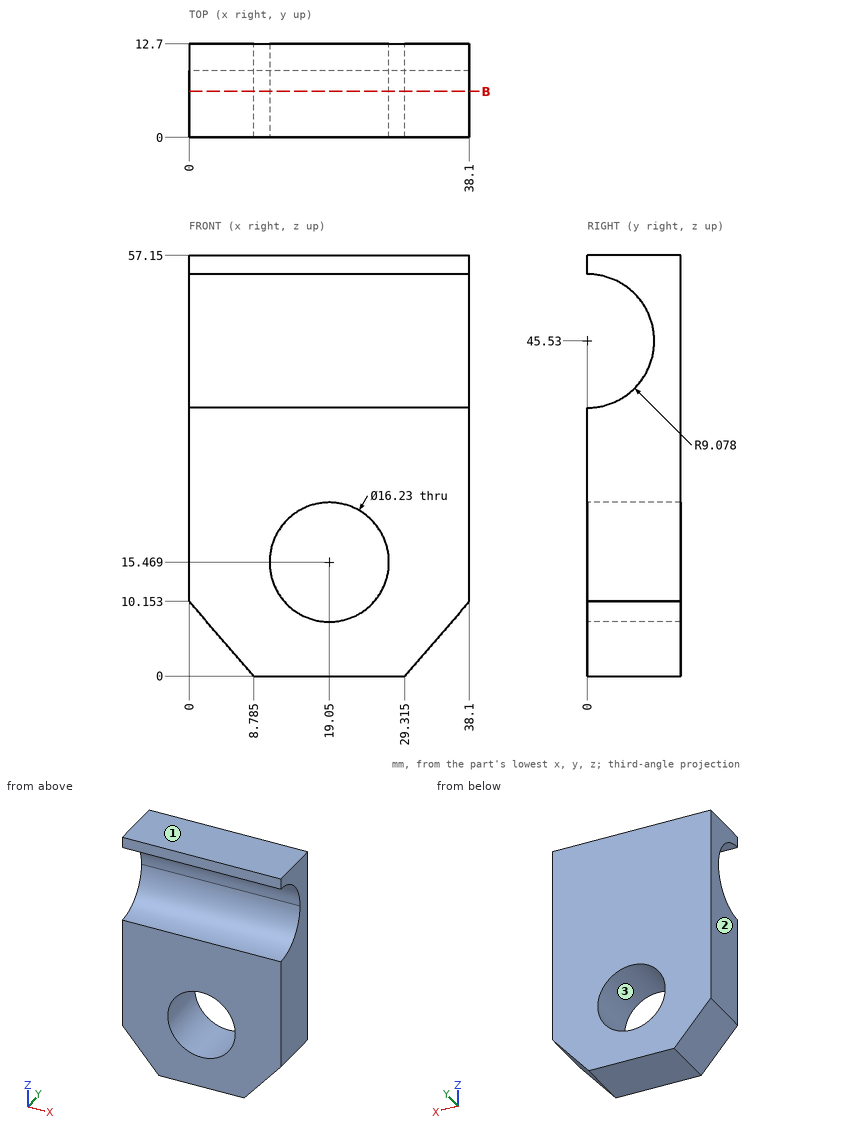
Can you work these out from the drawing? Everything is in mm from the part's minimum corner. Give positions to 0.01 mm unless a question says otherwise; leave off trailing zeros. Use a Markdown table: item, result. Add a question column.
1. I need wall thicknesses on probe 1 along X at (y, z) = (1.5, 15); probe 2 along X at (y, z) = (5, 21); probe 3 along Y at (x, z) = (34.5, 41.5) (1 decimal). Which ranges of each line are inside material? Lowest first, please. Write a range as from..to.
2. If we mould it in two halves opening along X, with no side actions, what happens to the marked faces 1, 2 and 3? For each: +X half, -X half, draft (parallel to the pull), parting line (faces both ways), or undercut.
3. Suppose I cut it at B-B (y = 6.25). Give the number of separate pieces and of enclosed holes in the cut face, and give its area (3 significant figures).
Results list:
| question | item | result |
|---|---|---|
| 1 | probe 1 | x = 0..10.95, 27.15..38.1 |
| 1 | probe 2 | x = 0..13.11, 24.99..38.1 |
| 1 | probe 3 | y = 8.1..12.7 |
| 2 | face 1 | draft |
| 2 | face 2 | -X half |
| 2 | face 3 | undercut |
| 3 | separate pieces | 2 |
| 3 | enclosed holes | 1 |
| 3 | area | 1,380 mm² |
